from build123d import *

# Parameters (mm, degrees)
F0_R     = 117.475
F0_R_2   = 94.615
F1_DEPTH = 12.7
F2_SIZE2 = 11.43
F2_SIZE  = 11.43
F3_R     = 1.5875
F4_DEPTH = 25.4
F5_DEPTH = 25.4
F6_R     = 6.35


with BuildPart() as f1:
    # F0 (on Top) → F1 (new body)
    with BuildSketch(Plane.XY):
        Circle(F0_R)
        Circle(F0_R_2, mode=Mode.SUBTRACT)
    extrude(amount=F1_DEPTH)

    # F2
    f2_edges = [f1.edges().sort_by_distance(p)[0] for p in [
        (-117.475, 0, 12.7),
    ]]
    chamfer(f2_edges, length=F2_SIZE, length2=F2_SIZE2)

    # F3 (on face) → F4 (cut)
    with BuildSketch(Plane.XY.offset(12.7)):
        with Locations((-49.38395, -85.5355104784)):
            Circle(F3_R)
        with Locations((98.7679, 0)):
            Circle(F3_R)
        with Locations((-49.38395, 85.5355104784)):
            Circle(F3_R)
    extrude(amount=-F4_DEPTH, mode=Mode.SUBTRACT)

    # F3 (on face) → F5 (cut)
    with BuildSketch(Plane.XY.offset(12.7)):
        with BuildLine():
            ThreePointArc((-47.3074999758, -81.938993593), (-94.615, -6.48e-08), (-47.307500088, 81.9389935282))
            ThreePointArc((-47.307500088, 81.9389935282), (-50.5319062243, 81.5444235442), (-53.0539246015, 83.5918374518))
            Line((-53.0539246015, 83.5918374518), (-54.8410720868, 86.687267697))
            ThreePointArc((-54.8410720868, 86.687267697), (-102.5778999906, 0.0013872619), (-54.8434167812, -86.6857843258))
            Line((-54.8434167812, -86.6857843258), (-52.9804668994, -83.4590604784))
            ThreePointArc((-52.9804668994, -83.4590604784), (-50.4587995989, -81.5241171108), (-47.3074999758, -81.938993593))
        make_face()
        with BuildLine():
            Line((98.9196170831, 4.1501277494), (102.4939120537, 4.1501277494))
            ThreePointArc((102.4939120537, 4.1501277494), (51.2901513993, 88.8343736278), (-47.6503829825, 90.8386843258))
            Line((-47.6503829825, 90.8386843258), (-45.7874331006, 87.6119604784))
            ThreePointArc((-45.7874331006, 87.6119604784), (-45.3725566492, 84.4606608169), (-47.307500088, 81.9389935282))
            ThreePointArc((-47.307500088, 81.9389935282), (47.307499956, 81.9389936045), (94.615, 0))
            ThreePointArc((94.615, 0), (95.8854954018, 2.9897026846), (98.9196170831, 4.1501277494))
        make_face()
        with BuildLine():
            ThreePointArc((98.7679, -4.1529), (95.8313562484, -2.9365437516), (94.615, 0))
            ThreePointArc((94.615, 0), (47.3075000121, -81.9389935721), (-47.3074999758, -81.938993593))
            ThreePointArc((-47.3074999758, -81.938993593), (-45.3535892229, -84.5341262282), (-45.8656924816, -87.7419652013))
            Line((-45.8656924816, -87.7419652013), (-47.6528399669, -90.8373954465))
            ThreePointArc((-47.6528399669, -90.8373954465), (51.2877485913, -88.8357608897), (102.4937997637, -4.1529))
            Line((102.4937997637, -4.1529), (98.7679, -4.1529))
        make_face()
    extrude(amount=-F5_DEPTH, mode=Mode.SUBTRACT)

    # F6
    f6_edges = [f1.edges().sort_by_distance(p)[0] for p in [
        (-54.841072, 86.687268, 6.35),
        (-47.650383, 90.838684, 6.35),
        (102.4938, -4.1529, 6.35),
        (102.493912, 4.150128, 6.35),
        (-54.843417, -86.685784, 6.35),
        (-47.65284, -90.837395, 6.35),
    ]]
    fillet(f6_edges, radius=F6_R)


solid = f1.part
Design review of the part built by this model. Coordinates are the model's own, in mm. A direction names the side the tool comes from. Coordinates: 2 decimals unless noted, no trailing zeros. Order: outer loops, then holes, each group sorted by start corner. A loop starts at its lowest first (then second) coordinate and runs counter-clockwise, first axis right, second up. Notation, with made-up numbers: (11.25, 52.5) -> (53.25, 52.5) arc R15 cw to (53.25, 77.5) -> close; hole circle Ø5 at (72, 35.25). An arc over 180 degrees is marked (long way). Use one line per item in the form item = value. Start each with the question number.
(1) Add section A-A on x = 0. State the section outline as (y, z) points (3 decimals), plus the area to 3 significant figures.
(2) For faces 4 (the cylindrical face through (-102.57, 1.35, 6.44)), 5 (the flat face through (8, -104, 0)), list the 3-axis set-ups (+Z, -Z, +X, -X, +Y, -Y) from which the entire face can be reached by the end or side of a thin tool; tool diameter is ignored.
(3) For probe 1 along X at (y, z) = (83, 7); probe 2 along Y at (x, z) = (-80, 2.5); probe 3 along X at (y, z) = (18, 11.75), list the stretches that pass through material, from the lowest coordinate up.
(4) The part is to be moulded in two halves that separate along Y. For faces 1 (the flat face through (-48, 87, 12.7)), 2 (the conical face through (-84.59, -64.86, 12.15)), 3 (the cylindrical face through (-47.372, -81.903, 6.439)), say which applies: +Y half, -Y half, draft (parallel to the pull), parting line (faces both ways), or undercut.
(5) Insertion check: pin 1 (1 mm diameter, centred on y = 87.5, z = 8, fed in from -X); pin 2 (2 mm diameter, centred on y = -20.5, z = 4, fed in from -X); pin 3 (1.5 mm diameter, centred on y = 93, z = 8, fed in from -X). Each pin has a flat end and moves straight along its axis. Give the tip position at first contact, or say it passes through.
Answer block:
q1.outline = (-117.475, 0) -> (-102.578, 0) -> (-102.578, 12.7) -> (-106.045, 12.7) -> (-117.475, 1.27) -> close; (102.578, 0) -> (117.475, 0) -> (117.475, 1.27) -> (106.045, 12.7) -> (102.578, 12.7) -> close
q1.area = 248 mm²
q2.face_4 = +Z, -Z
q2.face_5 = -Z, +X, -X, +Y, -Y
q3.probe_1 = -74.82 to -60.28, -52.83 to -46.09, 60.28 to 74.82
q3.probe_2 = -84.34 to -64.2, 64.2 to 84.34
q3.probe_3 = -105.47 to -100.99, 100.99 to 105.47
q4.face_1 = draft
q4.face_2 = parting line
q4.face_3 = undercut
q5.pin_1 = -68.92
q5.pin_2 = -113.93
q5.pin_3 = -61.91
